Source: CAD feature listing. Evaluate the final solid. Frame: model axes, mm. Face numbers are marked on the shaded views. A direction names the side the tool comes from. Coordinates: 2 decimals unless noted, no trailing zeros. Order: outer loops, then holes, each group sorted by start corner. A loop starts at its lowest first (then second) coordinate and runs counter-clockwise, first axis right, second up. Notation, with made-up numbers: (11.25, -8) - (52.25, -8) arc R16 cw to (52.25, 18) - close; hole circle Ø1 at (79, 74.25). An arc over 180 degrees is marked (long way). One line per question, with ' | ' between items. Start each with the question number.
(1) Draft query along Y for the marked faces 1, 2 and 3. Return one class per face: +Y half, -Y half, draft (parallel to the pull), parting line (faces both ways), or undercut.
(2) Section A-A (y = 0). Return the cut outline in (x, z), then the cut area to 3 significant figures.
(3) Access query for the marked faces 4 and 5. Directions: +Z, -Z, +X, -X, +Y, -Y. A direction counts if a zero-diameter tool reaches every point of the face in a straight line with its end or side. Return the directions, or none.
(4) Section B-B (z = 3.5). Return the cut outline in (x, y), then the cut area to 3 significant figures.
(5) Contact query for flat-ended pins moving along their axis: P1, Ø5, axis at y = 3, z = 1.5, coming from the +X side; P2, Ø5, axis at x = 4.5, y = -2, coming from the +Z side; P3, Ø2, axis at x = 7.5, z = 6.5, coming from the -Y side. Output: stop coordinate, or through.
(6) Line query: line 1 along Y through (x, z) = (0, 6.95); line 2 along Z through (x, y) = (9, 10.5); line 3 along X through (y, z) = (9, 7). Output: solid intervals per line, ascending.
(7) Section D-D (z = 0.5). Return the cut outline in (x, y).
from build123d import *

# Parameters (mm, degrees)
F0_R     = 16.5
F1_DEPTH = 3
F2_R     = 16.5
F2_R_2   = 15
F3_DEPTH = 6
F4_SIZE  = 2


with BuildPart() as f1:
    # F0 (on Top) → F1 (new body)
    with BuildSketch(Plane.XY):
        Circle(F0_R)
    extrude(amount=F1_DEPTH)

    # F2 (on face) → F3 (join)
    with BuildSketch(Plane.XY.offset(3)):
        Circle(F2_R)
        Circle(F2_R_2, mode=Mode.SUBTRACT)
    extrude(amount=F3_DEPTH)

    # F4
    f4_edges = [f1.edges().sort_by_distance(p)[0] for p in [
        (-16.5, 0, 0),
    ]]
    chamfer(f4_edges, length=F4_SIZE)


solid = f1.part
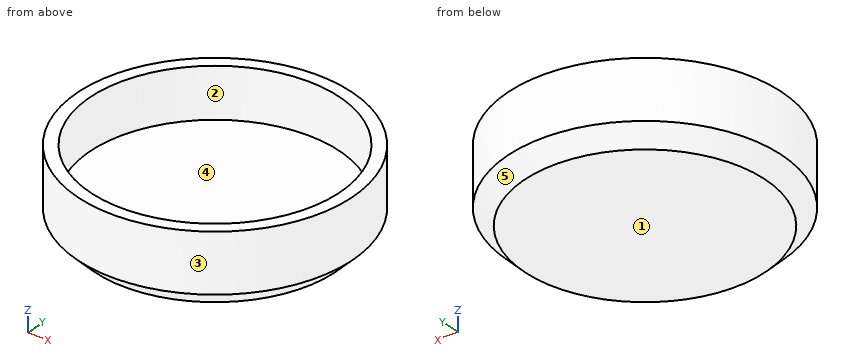
Response values:
1) face 1: draft | face 2: undercut | face 3: parting line
2) outline: (-16.5, 2) - (-14.5, 0) - (14.5, 0) - (16.5, 2) - (16.5, 9) - (15, 9) - (15, 3) - (-15, 3) - (-15, 9) - (-16.5, 9) - close | area: 113 mm²
3) face 4: +Z | face 5: -Z
4) outline: circle Ø33 at (0, 0); hole circle Ø30 at (0, 0) | area: 148 mm²
5) P1: stops at x = 16.49 | P2: stops at z = 3 | P3: stops at y = -15.17
6) line 1: y = -16.5 to -15, 15 to 16.5 | line 2: z = 0 to 3 | line 3: x = -13.83 to -12, 12 to 13.83
7) outline: circle Ø30 at (0, 0)
